Autodesk Inventor part; units mm, degrees
ref_plane "YZ Plane" through (0, 0, 0) normal (1, 0, 0) x (0, 1, 0)
ref_plane "XZ Plane" through (0, 0, 0) normal (0, 1, 0) x (-1, 0, 0)
ref_plane "XY Plane" through (0, 0, 0) normal (0, 0, 1) x (1, 0, 0)
sketch "Sketch1" plane through (0, 0, 0) normal (1, 0, 0) x (0, 1, 0)
  line L0 (0, 0) -> (10.1, 0)
  line L1 (10.1, 0) -> (10.1, -10)
  line L2 (10.1, -10) -> (0, -10)
  line L3 (0, -10) -> (0, 0)
  line L4 (10.1, 0) -> (15.65, 0)
  line L5 (15.65, 0) -> (15.65, -10)
  line L6 (15.65, -10) -> (10.1, -10)
  line L7 (10.1, -10) -> (10.1, 0)
  line L8 (0, 0) -> (-5.55, 0)
  line L9 (-5.55, 0) -> (-5.55, -10)
  line L10 (-5.55, -10) -> (0, -10)
  line L11 (0, -10) -> (0, 0)
  dimension "d0" = 10.1
  dimension "d1" = 10
  dimension "d2" = 5.55
  dimension "d3" = 5.55
extrude "Extrusion1" add sketch "Sketch1" along normal blind 2
extrude "Extrusion2" add sketch "Sketch1" against normal blind 2.8 contours L3 L10 L9 L8 | L4 L5 L6 L1
sketch "Sketch2" plane through (2, -5.55, 0) normal (0, 0, 1) x (1, 0, 0)
  line L0 (-4.8, 21.2) -> (0, 21.2)
  line L1 (0, 21.2) -> (-12, 21.2)
  line L2 (-12, 21.2) -> (-12, 23.2)
  line L3 (-12, 23.2) -> (0, 23.2)
  line L4 (0, 23.2) -> (0, 21.2)
  line L5 (0, 0) -> (0, 21.2)
  line L6 (0, 0) -> (-12, 0)
  line L7 (-12, 0) -> (-12, -2)
  line L8 (-12, -2) -> (0, -2)
  line L9 (0, -2) -> (0, 0)
  point P0 (-2, 5.55)
  dimension "d8" = 12
  dimension "d9" = 2
  dimension "d10" = 12
  dimension "d11" = 2
extrude "Extrusion3" add sketch "Sketch2" against normal blind 10
sketch "Sketch3" plane through (-10, 17.65, 0) normal (0, 1, 0) x (1, 0, 0)
  line L0 (0, 10) -> (7.2, 10)
  line L1 (0, 10) -> (3.2, 10)
  line L2 (3.2, 10) -> (3.2, 6.8)
  line L3 (3.2, 6.8) -> (0, 6.8)
  line L4 (0, 6.8) -> (0, 10)
  line L5 (3.2, 8.4) -> (2.2, 8.4)
  circle A0 centre (2.2, 8.4) radius 1
  point P0 (10, 0)
  dimension "d14" = 3.2
  dimension "d15" = 3.2
  dimension "d16" = 1
extrude "Extrusion4" cut sketch "Sketch3" against normal up to surface (25.2 mm away) contours A0
properties part number "measuring_support2"
Check sheet for the modelled part. Datum: model origin and axes. Units: mm. A direction names the side the tool comes from. Round coordinates to 2 decimals unless told otherwise and drop trailing zeros. Write each loop counter-clockwise with the first axis right and the second up, starting at its lowest first coordinate (ties: lowest second). Pieces come first, ordered by that corner, then holes. Notation, with made-up numbers: (-10, -7) -> (32, -7) arc R25 ccw to (32, 23) -> close; hole circle Ø11 at (-15, 8). An arc over 180 degrees is marked (long way). One line per question, with ' | ' between items. Start each with the question number.
1. Depth check by flat-ended pin: pin 1 (1.7 mm diameter, centred on y = -3, z = -7, fed in from -X); pin 2 (2.5 mm diameter, centred on x = -7.8, z = -8.4, fed in from +Y). Enter the tip coordinate at first touch or a pass-through.
2. Set-up check for faces 4 (the face through (0, 5, -5)), 5 (the face through (-4, -7.55, -5)): record each of +Z, -Z, +X, -X, +Y, -Y from which the full face is reachable in a straight line by a thin tool's end or side.
3. Release check for a two-part mould opening along X. For faces 1 (the face through (2, 5, -5)), 2 (the face through (-10, 17, -5)), 3 (the face through (-6.876, 16.664, -8.017)) record: +X half, -X half, draft (parallel to the pull), parting line (faces both ways), or undercut.
4. Sectioned sample at C-C, the plane x = -1.5. Record the cut outline in (y, z), then the cut area to 3 significant figures.
5. Scan lines: line 1 along Z through (x, y) = (-7.8, -6.05); line 2 along Y through (x, z) = (-3.25, -7.75); line 3 along X through (y, z) = (17, -8.4). Record each from-to range of solid material in increasing order. Write a range as from..to.
6. Sectioned sample at B-B, the plane x = -7.8. Record the cut outline in (y, z).
7. Sectioned sample at A-A, the plane z = -8.4. Record the cut outline in (x, y), then the cut area to 3 significant figures.
8. Sectioned sample at D-D, the plane z = -6. Record the cut outline in (x, y).
Taken from the geometry:
1) pin 1: stops at x = -2.8 | pin 2: stops at y = 17.65
2) face 4: +Z, -Z, -X | face 5: +Z, -Z, +X, -X, -Y
3) face 1: +X half | face 2: -X half | face 3: undercut
4) outline: (-7.55, -10) -> (0, -10) -> (0, 0) -> (-7.55, 0) -> close; (10.1, -10) -> (17.65, -10) -> (17.65, 0) -> (10.1, 0) -> close | area: 151 mm^2
5) line 1: z = -10..-9.4, -7.4..0 | line 2: y = -7.55..-5.55, 15.65..17.65 | line 3: x = -10..-8.8, -6.8..2
6) outline: (-7.55, -10) -> (-5.55, -10) -> (-5.55, -9.4) -> (-7.55, -9.4) -> close; (-7.55, -7.4) -> (-5.55, -7.4) -> (-5.55, 0) -> (-7.55, 0) -> close; (15.65, -10) -> (17.65, -10) -> (17.65, -9.4) -> (15.65, -9.4) -> close; (15.65, -7.4) -> (17.65, -7.4) -> (17.65, 0) -> (15.65, 0) -> close
7) outline: (-10, -7.55) -> (-8.8, -7.55) -> (-8.8, -5.55) -> (-10, -5.55) -> close; (-10, 15.65) -> (-8.8, 15.65) -> (-8.8, 17.65) -> (-10, 17.65) -> close; (-6.8, -7.55) -> (2, -7.55) -> (2, 17.65) -> (-6.8, 17.65) -> (-6.8, 15.65) -> (-2.8, 15.65) -> (-2.8, 10.1) -> (0, 10.1) -> (0, 0) -> (-2.8, 0) -> (-2.8, -5.55) -> (-6.8, -5.55) -> close | area: 113 mm^2
8) outline: (-10, -7.55) -> (2, -7.55) -> (2, 17.65) -> (-10, 17.65) -> (-10, 15.65) -> (-2.8, 15.65) -> (-2.8, 10.1) -> (0, 10.1) -> (0, 0) -> (-2.8, 0) -> (-2.8, -5.55) -> (-10, -5.55) -> close
